CAD build for the part. Positions are in the model's coordinates, mm. A direction names the side the tool comes from. Coordinates: 2 decimals unless noted, no trailing zeros. Order: outer loops, then holes, each group sorted by start corner. A loop starts at its lowest first (then second) coordinate and runs counter-clockwise, first axis right, second up. Notation, with made-up numbers: (-7.5, 48) - (16.5, 48) arc R20 cw to (16.5, 80) - close; hole circle Ø9 at (42, -22.5). An arc over 180 degrees is marked (long way). Return JSON: item names as keys, results as strings.
from build123d import *

# Parameters (mm, degrees)
F1_DEPTH = 12.7


with BuildPart() as f1:
    # F0 (on Front) → F1 (new body)
    with BuildSketch(Plane.XZ):
        Polygon((-26.490386, 45.168456), (-35.56, 36.278456), (-3.277726, 3.343949), (-3.277726, 12.044498), (-3.277726, 21.486806), align=None)
        Polygon((-3.277726, 12.044498), (-3.277726, 3.343949), (0, 0), (2.550656, 2.602189), (2.550656, 12.044498), align=None)
        Polygon((2.550656, 12.044498), (2.550656, 2.602189), (35.56, 36.278456), (26.490386, 45.168456), (2.550656, 21.486806), align=None)
    extrude(amount=F1_DEPTH)


solid = f1.part
Item 1: Mould opens along X. For faces 1 (the flat face through (31.09, -6.26, 40.66)), 2 (the flat face through (-30.96, -6.26, 40.79)), 3 (the flat face through (-14.72, -6.26, 33.16)) say: released by +X, released by -X, zero draft, split by the parting line, or undercut.
Findings below:
{"face 1": "released by +X", "face 2": "released by -X", "face 3": "undercut"}
Item 2: Which spindle directions (+Z, -Z, +X, -X, +Y, -Y) get a long thin tool onto all of the face, cutting with end or side? Do faces 4 (the flat face through (2.551, -6, 17)), 5 (the flat face through (-5, -12.7, 23)). Say none if no direction does.
Findings below:
{"face 4": "+Z, +Y, -Y", "face 5": "+Z, -Z, +X, -X, -Y"}
Item 3: Band-saw the part on D-D, the plane x = 10.5. List the corners of the cut face in (y, z), then the cut area to 3 significant figures.
Findings below:
{"outline": "(-12.7, 10.71) - (0, 10.71) - (0, 29.35) - (-12.7, 29.35) - close", "area": "237 mm²"}
Item 4: Band-saw the part on B-B, the plane z = 27.5. List the corners of the cut face in (x, y).
Findings below:
{"outline": "(-26.96, -12.7) - (-9.17, -12.7) - (-9.17, 0) - (-26.96, 0) - close; (8.63, -12.7) - (26.96, -12.7) - (26.96, 0) - (8.63, 0) - close"}
Item 5: Wall check: L1, parallel to X at y = -8.5, z = 29; L2, parallel to X at y = -6.5, z = 42.5; L3, parallel to Z at x = -25.5, y = -0.5. Give the ranges that are in metal, low to high. Write a range as [from, to].
Findings below:
{"L1": "x = [-28.43, -10.64], [10.15, 28.43]", "L2": "x = [-29.21, -23.87], [23.79, 29.21]", "L3": "z = [26.02, 44.16]"}
Item 6: Band-saw the part on A-A, the plane y = -11.75. List the corners of the cut face in (x, z).
Findings below:
{"outline": "(-35.56, 36.28) - (0, 0) - (2.55, 2.6) - (35.56, 36.28) - (26.49, 45.17) - (2.55, 21.49) - (2.55, 12.04) - (-3.28, 12.04) - (-3.28, 21.49) - (-26.49, 45.17) - close"}
Item 7: Drop flat-ended pins along their axis: P1, Ø7.5, axis at y = -3.5, z = 15, coming from the -X side; P2, Ø5, axis at x = 15.5, y = -4, coming from the -Z side; P3, Ø5, axis at x = -2.5, y = -4.5, coming from the +Z side. Give the stop position or say it passes through.
Findings below:
{"P1": "stops at x = -18.38", "P2": "stops at z = 13.26", "P3": "stops at z = 23.24"}
Item 8: Band-saw the part on C-C, the plane z = 16.5. List the corners of the cut face in (x, y).
Findings below:
{"outline": "(-16.17, -12.7) - (-3.28, -12.7) - (-3.28, 0) - (-16.17, 0) - close; (2.55, -12.7) - (16.17, -12.7) - (16.17, 0) - (2.55, 0) - close"}
